```python
from build123d import *

# Parameters (mm, degrees)
SKETCH2_R           = 1
BOSS_EXTRUDE4_DEPTH = 30
FILLET2_R           = 1
ESCALA1_SCALE       = 0.5


with BuildPart() as part:
    # Sketch2 → Boss-Extrude4 (new body)
    with BuildSketch(Plane.XY):
        Circle(SKETCH2_R)
    extrude(amount=BOSS_EXTRUDE4_DEPTH)

    # Fillet2
    fillet2_edges = [part.edges().sort_by_distance(p)[0] for p in [
        (-1, 0, 0),
        (-1, 0, 30),
    ]]
    fillet(fillet2_edges, radius=FILLET2_R)


with BuildPart() as part_1:
    # Escala1: scaled about (0, 0, 15)
    add(part.part.scale(ESCALA1_SCALE).moved(Location((0, 0, 7.5))))


solid = part_1.part
```
Source: CAD feature listing. Evaluate the final solid. Frame: model axes, mm. Coordinates: 2 decimals unless noted, no trailing zeros. Write each loop counter-clockwise with the first axis right and the second up, starting at its lowest first coordinate (ties: lowest second). Pieces come first, ordered by that corner, then holes. Notation, with made-up numbers: (24, 61) - (45, 61) arc R37 ccw to (45, 97) - close; hole circle Ø10 at (-25, 51.25). An arc over 180 degrees is marked (long way). Answer as a JSON object with one key per item and string values.
Q1. Section query A-A, the plane x = 0.3. Output: boundary loops of the cut face in (y, z), plus the area to 3 significant figures.
Ans:
{"outline": "(-0.4, 8) arc R0.4 ccw to (0.4, 8) - (0.4, 22) arc R0.4 ccw to (-0.4, 22) - close", "area": "11.7 mm2"}
Q2. Material intervals for line 1 (Z direction, x = -0.2, y = 0.35); line 2 (Y direction, x = -0.25, z = 18.75); line 3 (X direction, y = -0.15, z = 13.25), sorted ascending. Write a range as [from, to].
Ans:
{"line 1": "z = [7.7, 22.3]", "line 2": "y = [-0.43, 0.43]", "line 3": "x = [-0.48, 0.48]"}
Q3. Section query B-B, the plane z = 16. Output: boundary loops of the cut face in (x, y).
Ans:
{"outline": "circle Ø1 at (0, 0)"}
Q4. Section query C-C, the plane y = 0.2. Output: boundary loops of the cut face in (x, z).
Ans:
{"outline": "(-0.46, 8) arc R0.46 ccw to (0.46, 8) - (0.46, 22) arc R0.46 ccw to (-0.46, 22) - close"}
